Model file for the job. Use its own axes, mm. Face numbers are marked on the shaded views. A direction names the side the tool comes from. Coordinates: 2 decimals unless noted, no trailing zeros. Write each loop counter-clockwise with the first axis right and the second up, starting at its lowest first coordinate (ties: lowest second). Pieces come first, ordered by that corner, then holes. Notation, with made-up numbers: (23.5, -16) - (61.5, -16) arc R28 cw to (61.5, 5) - close; hole circle Ø6 at (-20, 39). An arc over 180 degrees is marked (long way). Put each result on its own line as item: value. Start each with the question number.
1. Saw through at C-C, the plane z = 5. Write the cut outline in (x, y) (3 decimals).
2. Drill centre lines: L1, parallel to Y at x = 0, z = 9 (3 decimals); L2, parallel to Y at x = 0, z = -4.75 (3 decimals); L3, parallel to Z at x = -36.5, y = 32 (3 decimals). Where is each one in solid material? Low to high. Write a range as from..to.
3. Saw through at A-A, the plane x = 0. Write the cut outline in (y, z) (3 decimals).
4. Saw through at D-D, the plane x = -25. Write the cut outline in (y, z) (3 decimals).
5. Drop flat-ended pins along their axis: P1, Ø5, axis at x = 13.5, z = 7, coming from the +Y side; P2, Ø10, axis at x = -45.5, y = 1.5, coming from the -Z side; P3, Ø4, axis at y = -16, z = -6, coming from the -X side. Give the stop position or say it passes through.
6. Pull direction X, two halves, no side cores. Call the marked faces 4, 5 and 6: released by +X, released by -X, zero draft, split by the parting line, or undercut.
7. Which spindle directions (+Z, -Z, +X, -X, +Y, -Y) get a long thin tool onto all of the face, cutting with end or side? Do the marked faces 1, 2 and 3. Say none if no direction does.
```python
from build123d import *

# Parameters (mm, degrees)
F0_R     = 59.69
F0_R_2   = 56.515
F1_DEPTH = 12.7
F2_DEPTH = 3.175
F3_R     = 21.425
F3_R_2   = 18.25
F4_DEPTH = 12.7


# Not quite as in the source:
# - a feature names something its author has since deleted; it is built from what else it names


with BuildPart() as f1:
    # F0 (on Top) → F1 (new body)
    with BuildSketch(Plane.XY):
        Circle(F0_R)
        Circle(F0_R_2, mode=Mode.SUBTRACT)
    extrude(amount=F1_DEPTH)

    # F0 (on Top) → F2 (join)
    with BuildSketch(Plane.XY):
        Circle(F0_R_2)
    extrude(amount=F2_DEPTH)

    # F3 (on face) → F4 (join)
    with BuildSketch(Plane.XY):
        Circle(F3_R)
        Circle(F3_R_2, mode=Mode.SUBTRACT)
    extrude(amount=-F4_DEPTH)


solid = f1.part
```
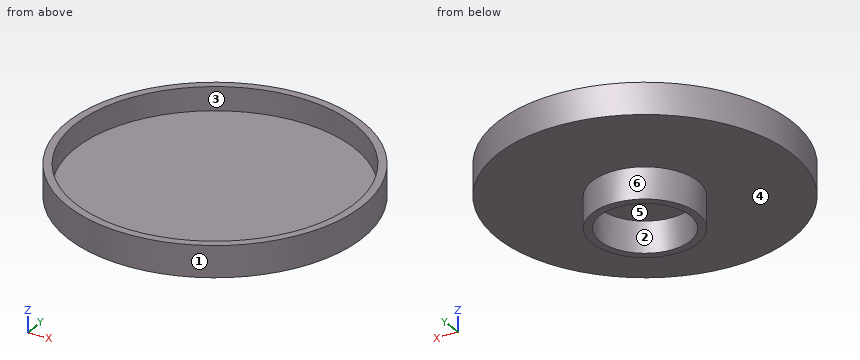
Final values:
1. outline: circle Ø119.38 at (0, 0); hole circle Ø113.03 at (0, 0)
2. L1: y = -59.69..-56.515, 56.515..59.69
2. L2: y = -21.425..-18.25, 18.25..21.425
2. L3: z = 0..3.175
3. outline: (-59.69, 0) - (-21.425, 0) - (-21.425, -12.7) - (-18.25, -12.7) - (-18.25, 0) - (18.25, 0) - (18.25, -12.7) - (21.425, -12.7) - (21.425, 0) - (59.69, 0) - (59.69, 12.7) - (56.515, 12.7) - (56.515, 3.175) - (-56.515, 3.175) - (-56.515, 12.7) - (-59.69, 12.7) - close
4. outline: (-54.202, 0) - (54.202, 0) - (54.202, 12.7) - (50.685, 12.7) - (50.685, 3.175) - (-50.685, 3.175) - (-50.685, 12.7) - (-54.202, 12.7) - close
5. P1: stops at y = 58.67
5. P2: stops at z = 0
5. P3: stops at x = -16.22
6. face 4: zero draft
6. face 5: undercut
6. face 6: split by the parting line
7. face 1: +Z, -Z
7. face 2: -Z
7. face 3: +Z
